Autodesk Inventor part; units mm, degrees
ref_plane "YZ Plane" through (0, 0, 0) normal (1, 0, 0) x (0, 1, 0)
ref_plane "XZ Plane" through (0, 0, 0) normal (0, 1, 0) x (-1, 0, 0)
ref_plane "XY Plane" through (0, 0, 0) normal (0, 0, 1) x (1, 0, 0)
sketch "Sketch1" plane through (0, 0, 0) normal (1, 0, 0) x (0, 1, 0)
  line L0 (0, 0) -> (0, -2)
  line L1 (0, -2) -> (45, -2)
  line L2 (45, -2) -> (45, -5)
  line L3 (45, -5) -> (0, -5)
  line L4 (0, 0) -> (47, 0)
  line L5 (47, 0) -> (47, -7)
  line L6 (47, -7) -> (0, -7)
  line L7 (0, -7) -> (0, -5)
  circle A0 centre (1.5, -2) radius 1.5
  point P0 (3, -2)
  point P1 (32, -2)
  point P2 (32, -5)
  dimension "d0" = 2
  dimension "d1" = 45
  dimension "d2" = 3
  dimension "d3" = 47
  dimension "d4" = 7
  dimension "d5" = 3
  dimension "d6" = 1.5
extrude "Extrusion1" add sketch "Sketch1" along normal blind 56
sketch "Sketch3" plane through (0, 0, 0) normal (0, 1, 0) x (-1, 0, 0)
  line L0 (0, -7) -> (-56, -7)
  line L1 (-34.7, -7) -> (-21.3, -7)
  line L2 (-21.3, -7) -> (-18.5, -9.8)
  line L3 (-18.5, -9.8) -> (-37.5, -9.8)
  line L4 (-34.7, -7) -> (-37.5, -9.8)
  line L5 (-56, -5) -> (-56, -7)
  point P0 (0, 0)
  point P1 (-28, -7)
  point P2 (-56, -6)
  point P3 (-21.3, -7)
  dimension "d10" = 135
  dimension "d11" = 135
  dimension "d12" = 2.8
  dimension "d13" = 28
  dimension "d14" = 19
extrude "Extrusion2" add sketch "Sketch3" along normal blind 30
fillet "Rundung1" radius 2 8 edges at (56, 47, -3.5) (56, 0, -6) (0, 47, -3.5) (0, 0, -6) (0, 23.5, 0) (28, 47, 0) (56, 23.5, 0) (28, 0, 0)
properties part number "belt_clip"
For this review, take the finished solid that the model builds, in its own axes (mm). A direction names the side the tool comes from. Coordinates: 2 decimals unless noted, no trailing zeros. Answer as a JSON object with one key per item and string values. Group by question number.
1. For probe 1 along Z at (x, y) = (30.5, 31.5); probe 2 along Z at (x, y) = (21.5, 14.5); probe 3 along Y at (x, z) = (35, -7.5), list the stretches that pass through material, from the lowest coordinate up.
2. The part is to be moulded in two halves that separate along Y. For faces 1 (the flat face through (28, 47, -4)), 2 (the flat face through (28, 0, -7)), 3 (the flat face through (0, 22, -6)), 4 (the flat face through (28, 24, -2)), say which applies: pulls with the +Y half, pulls with the -Y half, needs draft (parallel to the pull), parting line crosses it, or undercut.
3. Clearance check with flat-ended pins moving along their axes: P1, Ø2.5, axis at x = 37.5, z = -3.5, coming from the -Y side; P2, Ø2, axis at x = 30, z = -9, coming from the +Y side. State where each tip first meets the part, or that it passes through.
4. For faces 5 (the flat face through (28, 30, -8)), 6 (the flat face through (28, 23, -5)), 7 (the cylindrical face through (0.57, 0.6, -5.99)), 8 (the cylindrical face through (27.6, 1.5, -3.5)), list the 3-axis set-ups (+Z, -Z, +X, -X, +Y, -Y) from which the entire face can be reached by the end or side of a thin tool; tool diameter is ignored.
Final values:
{
 "1": {"probe 1": "-7 to -5, -2 to 0", "probe 2": "-9.8 to -5, -2 to 0", "probe 3": "0 to 30"},
 "2": {"face 1": "pulls with the +Y half", "face 2": "pulls with the -Y half", "face 3": "needs draft", "face 4": "undercut"},
 "3": {"P1": "y = 0.02", "P2": "y = 30"},
 "4": {"face 5": "-Z, +X, -X, +Y", "face 6": "+X, -X, -Y", "face 7": "-Z, -X, -Y", "face 8": "+X, -X"}
}
